Check sheet for the modelled part. Datum: model origin and axes. Units: mm. A direction names the side the tool comes from. Coordinates: 2 decimals unless noted, no trailing zeros. Write each loop counter-clockwise with the first axis right and the second up, starting at its lowest first coordinate (ties: lowest second). Pieces come first, ordered by that corner, then holes. Notation, with made-up numbers: (-25, -4.5) - (-13, -4.5) arc R19 cw to (-13, 31.5) - close; hole circle Ø4 at (-35.75, -37). An arc over 180 degrees is marked (long way). Answer as CSV lines item,"result". Start each with the question number.
from build123d import *

# Parameters (mm, degrees)
SALIENTE_EXTRUIR1_DEPTH = 7.05
CROQUIS1_3_R            = 3.5
SALIENTE_EXTRUIR2_DEPTH = 0.75
CROQUIS2_R              = 1.2
SALIENTE_EXTRUIR3_DEPTH = 2.4
CROQUIS3_R              = 1
SALIENTE_EXTRUIR4_DEPTH = 1.2
CORTAR_EXTRUIR1_REACH   = 16.574
SALIENTE_EXTRUIR5_DEPTH = 0.7
SALIENTE_EXTRUIR6_DEPTH = 4.8
CORTAR_EXTRUIR2_DEPTH   = 4.8
CORTAR_EXTRUIR4_DEPTH   = 4.8


# Read off the part's stored shape, not the designer's step: Simetr_a1
with BuildPart() as part:
    # Croquis1 → Saliente-Extruir1 (new, symmetric)
    with BuildSketch(Plane(origin=(0, 0, 0), x_dir=(0, 0, -1), z_dir=(1, 0, 0))):
        with BuildLine():
            ThreePointArc((-2.343074903, -2.1), (0, -1.2), (2.343074903, -2.1))
            Line((2.343074903, -2.1), (3.9, -2.1))
            Line((3.9, -2.1), (3.9, 0))
            Line((3.9, 0), (-3.9, 0))
            Line((-3.9, 0), (-3.9, -2.1))
            Line((-3.9, -2.1), (-2.343074903, -2.1))
        make_face()
    extrude(amount=SALIENTE_EXTRUIR1_DEPTH, both=True)

    # Croquis1_3 → Saliente-Extruir2 (add, symmetric)
    with BuildSketch(Plane(origin=(0, 0, 0), x_dir=(0, 0, -1), z_dir=(1, 0, 0))):
        with Locations((0, -4.7)):
            Circle(CROQUIS1_3_R)
    extrude(amount=SALIENTE_EXTRUIR2_DEPTH, both=True)

    # Croquis2 → Saliente-Extruir3 (add)
    with BuildSketch(Plane(origin=(0.75, 0, 0), x_dir=(0, 0, -1), z_dir=(1, 0, 0))):
        with Locations((0, -4.7)):
            Circle(CROQUIS2_R)
    extrude(amount=SALIENTE_EXTRUIR3_DEPTH)

    # Croquis3 → Saliente-Extruir4 (add)
    with BuildSketch(Plane(origin=(3.15, 0, 0), x_dir=(0, 0, -1), z_dir=(1, 0, 0))):
        with Locations((0, -4.7)):
            Circle(CROQUIS3_R)
    extrude(amount=SALIENTE_EXTRUIR4_DEPTH)

    # Croquis4 → Cortar-Extruir1 (cut, up to next)
    with BuildSketch(Plane(origin=(4.35, 0, 0), x_dir=(0, 0, -1), z_dir=(1, 0, 0)), mode=Mode.PRIVATE) as cortar_extruir1_sk1:
        with BuildLine():
            Line((-0.661437828, -3.95), (0.661437828, -3.95))
            ThreePointArc((0.661437828, -3.95), (0, -3.7), (-0.661437828, -3.95))
        make_face()
    cortar_extruir1_tool1 = extrude(cortar_extruir1_sk1.sketch, amount=-CORTAR_EXTRUIR1_REACH, mode=Mode.PRIVATE) & part.part
    add(cortar_extruir1_tool1.solids().sort_by_distance((4.35, -3.848845, 0))[0], mode=Mode.SUBTRACT)

    # Croquis5 → Saliente-Extruir5 (add)
    with BuildSketch(Plane(origin=(3.15, 0, 0), x_dir=(0, 0, -1), z_dir=(1, 0, 0))):
        with BuildLine():
            ThreePointArc((0.7, -5.414142843), (0, -5.7), (-0.7, -5.414142843))
            Line((-0.7, -5.414142843), (-0.7, -5.794142843))
            ThreePointArc((-0.7, -5.794142843), (0, -5.99890283), (0.7, -5.794142843))
            Line((0.7, -5.794142843), (0.7, -5.414142843))
        make_face()
    extrude(amount=SALIENTE_EXTRUIR5_DEPTH)

    # Croquis6 → Saliente-Extruir6 (add)
    with BuildSketch(Plane(origin=(0, 0, 0), x_dir=(1, 0, 0), z_dir=(0, 1, 0))):
        with BuildLine():
            Line((2.75, -2.4), (5.15, -2.4))
            ThreePointArc((5.15, -2.4), (5.547451294, -1.597451294), (6.35, -1.2))
            Line((6.35, -1.2), (6.35, 1.2))
            ThreePointArc((6.35, 1.2), (5.547451294, 1.597451294), (5.15, 2.4))
            Line((5.15, 2.4), (2.75, 2.4))
            ThreePointArc((2.75, 2.4), (2.352548706, 1.597451294), (1.55, 1.2))
            Line((1.55, 1.2), (1.55, -1.2))
            ThreePointArc((1.55, -1.2), (2.352548706, -1.597451294), (2.75, -2.4))
        make_face()
    extrude(amount=SALIENTE_EXTRUIR6_DEPTH)

    # Croquis7 → Cortar-Extruir2 (cut)
    with BuildSketch(Plane(origin=(0, 4.8, 0), x_dir=(1, 0, 0), z_dir=(0, 1, 0))):
        with BuildLine():
            Line((3.323900966, -1.252198067), (4.576099034, 1.252198067))
            ThreePointArc((4.576099034, 1.252198067), (2.697801933, 0.626099034), (3.323900966, -1.252198067))
        make_face()
        with BuildLine():
            ThreePointArc((5.05, 0.866025404), (4.834384984, 1.085294062), (4.576099034, 1.252198067))
            Line((4.576099034, 1.252198067), (3.323900966, -1.252198067))
            ThreePointArc((3.323900966, -1.252198067), (4.255659718, -1.366225507), (5.05, -0.866025404))
            Line((5.05, -0.866025404), (5.05, 0.866025404))
        make_face()
    extrude(amount=-CORTAR_EXTRUIR2_DEPTH, mode=Mode.SUBTRACT)

    # Croquis8 → Cortar-Extruir4 (cut)
    with BuildSketch(Plane.XY.offset(2.4)):
        Polygon((5.85, 4.8), (6.35, 1.8), (6.35, 4.8), align=None)
    extrude(amount=-CORTAR_EXTRUIR4_DEPTH, mode=Mode.SUBTRACT)

    # Simetr_a1: part across plane


with BuildPart() as part_1:
    add(part.part)
    add(part.part.mirror(Plane(origin=(0, 0, 0), x_dir=(0, 0, 1), z_dir=(1, 0, 0))))


solid = part_1.part
(1) Go/stop test with flat-tipped pins: P1, Ø1.5, axis at x = 4, z = 0.5, coming from the -Y side; P2, Ø1.4, axis at y = 1, z = 0.5, coming from the +X side; P3, Ø1.5, axis at x = -5.5, z = -1.5, coming from the -Y side. Record where each tip stops, or that it passes through.
(2) Material ranges on probe 1 along X at (y, z) = (2.75, -1); probe 2 along Z at (x, y) = (-4.75, 0.5); probe 3 along X at (y, z) = (3, 0.75), recorded low to high. Write a range as from..to.
(3) Cross-section at B-B on y = 3.25. Record the boundary of the cut face in (x, z).
(4) Cross-section at A-A on x = 1. Record the boundary of the cut face in (y, z).
(5) Cross-section at D-D on x = -5.5. Record the boundary of the cut face in (y, z), plus the area to 3 significant figures.
(6) Tool access check on faces 1 (the face through (-5.05, 2, 0)), 2 (the face through (1.55, 2, 0)), 3 (the face through (4, -5.7, 0)). Record the directions out of +Z, -Z, +X, -X, +Y, -Y that give a thin tool (end or side, any length) a straight path to the whole face; none if there is none.
(7) Release check for a two-part mould opening along Z. For faces 4 (the face through (0, 0, 0)), 5 (the face through (3.9, -1.2, 0)), 6 (the face through (-4, 2, -2.4)) record: pulls with the +Z half, pulls with the -Z half, needs draft (parallel to the pull), parting line crosses it, or undercut.
(8) Cross-section at C-C on y = -4.7. Record the boundary of the cut face in (x, z), plus the area to 3 significant figures.
Checked values:
1,P1,"y = -6"
1,P2,"x = 6.35"
1,P3,"y = -2.02"
2,probe 1,"-6.19..-4.93, -2.97..-1.55, 1.55..2.97, 4.93..6.19"
2,probe 2,"-2.4..-1.15, 1.15..2.4"
2,probe 3,"-6.15..-5.05, -2.77..-1.55, 1.55..2.77, 5.05..6.15"
3,outline,"(-6.11, -1.25) arc R1.4 cw to (-5.15, -2.4) - (-2.75, -2.4) arc R1.4 cw to (-1.55, -1.2) - (-1.55, 1.2) arc R1.4 cw to (-2.75, 2.4) - (-5.15, 2.4) arc R1.4 cw to (-6.11, 1.25) - close; (1.55, -1.2) arc R1.4 cw to (2.75, -2.4) - (5.15, -2.4) arc R1.4 cw to (6.11, -1.25) - (6.11, 1.25) arc R1.4 cw to (5.15, 2.4) - (2.75, 2.4) arc R1.4 cw to (1.55, 1.2) - close; hole (-5.05, -0.87) arc R1.4 ccw (long way) to (-5.05, 0.87) - close; hole (5.05, -0.87) - (5.05, 0.87) arc R1.4 ccw (long way) to start"
4,outline,"circle Ø2.4 at (-4.7, 0); (-2.1, -3.9) - (0, -3.9) - (0, 3.9) - (-2.1, 3.9) - (-2.1, 2.34) arc R3.5 cw to (-2.1, -2.34) - close; hole (-3.95, -0.66) arc R1 ccw to (-3.95, 0.66) - close"
5,outline,"(-2.1, -3.9) - (0, -3.9) - (0, -1.65) - (4.8, -1.65) - (4.8, 1.65) - (0, 1.65) - (0, 3.9) - (-2.1, 3.9) - (-2.1, 2.34) arc R3.5 cw to (-2.1, -2.34) - close"
5,area,"29.3 mm^2"
6,face 1,"+Y"
6,face 2,"+Z, -Z, +Y"
6,face 3,"+X"
7,face 4,"needs draft"
7,face 5,"undercut"
7,face 6,"pulls with the -Z half"
8,outline,"(-4.35, -1) - (-3.15, -1) - (-3.15, -1.2) - (-0.75, -1.2) - (-0.75, -3.5) - (0.75, -3.5) - (0.75, -1.2) - (3.15, -1.2) - (3.15, -1) - (4.35, -1) - (4.35, 1) - (3.15, 1) - (3.15, 1.2) - (0.75, 1.2) - (0.75, 3.5) - (-0.75, 3.5) - (-0.75, 1.2) - (-3.15, 1.2) - (-3.15, 1) - (-4.35, 1) - close"
8,area,"26.8 mm^2"
